from build123d import *

# Parameters (mm, degrees)
SKETCH1_W           = 47
SKETCH1_H           = 47
BOSS_EXTRUDE1_DEPTH = 30
SKETCH2_W           = 43.5
SKETCH2_H           = 43.5
CUT_EXTRUDE1_DEPTH  = 26.1
SKETCH5_W           = 47
SKETCH5_H           = 47
BOSS_EXTRUDE3_DEPTH = 3
CUT_EXTRUDE3_REACH  = 62.508
SKETCH4_W           = 2
SKETCH4_H           = 20
LPATTERN1_COUNT     = 7
LPATTERN1_PITCH     = 4
SKETCH8_W           = 26
SKETCH8_H           = 2
BOSS_EXTRUDE4_DEPTH = 2
LPATTERN2_COUNT     = 5
LPATTERN2_PITCH     = 4
SKETCH9_W           = 18
SKETCH9_H           = 9.389923451
CUT_EXTRUDE4_DEPTH  = 10
SKETCH10_W          = 15
SKETCH10_H          = 10
CUT_EXTRUDE5_DEPTH  = 61.508263898
SKETCH11_W          = 9.504801384
SKETCH11_H          = 14.465733587
SKETCH11_W_2        = 14.602344504
SKETCH11_H_2        = 6.519720082
CUT_EXTRUDE6_DEPTH  = 47.834816109


with BuildPart() as part:
    # Sketch1 → Boss-Extrude1 (new body)
    with BuildSketch(Plane(origin=(0, 0, 0), x_dir=(1, 0, 0), z_dir=(0, 1, 0))):
        Rectangle(SKETCH1_W, SKETCH1_H)
    extrude(amount=BOSS_EXTRUDE1_DEPTH)

    # Sketch2 → Cut-Extrude1 (cut)
    with BuildSketch(Plane.XZ):
        Rectangle(SKETCH2_W, SKETCH2_H)
    extrude(amount=-CUT_EXTRUDE1_DEPTH, mode=Mode.SUBTRACT)

    # Sketch5 → Boss-Extrude3 (add)
    with BuildSketch(Plane.XZ):
        Rectangle(SKETCH5_W, SKETCH5_H)
        Polygon((-16.6, 21.75), (-21.75, 21.75), (-21.75, 16.6), (-21.75, -16.6), (-21.75, -21.75), (-16.6, -21.75), (16.6, -21.75), (21.75, -21.75), (21.75, -16.6), (21.75, 16.6), (21.75, 21.75), (16.6, 21.75), align=None, mode=Mode.SUBTRACT)
    extrude(amount=BOSS_EXTRUDE3_DEPTH)

    # Sketch4 → Cut-Extrude3 (cut, up to next)
    with BuildSketch(Plane(origin=(0, 0, -23.5), x_dir=(-1, 0, 0), z_dir=(0, 0, -1)), mode=Mode.PRIVATE) as cut_extrude3_sk1:
        with Locations((-12, 13.157296847)):
            Rectangle(SKETCH4_W, SKETCH4_H)
    cut_extrude3_tool1 = extrude(cut_extrude3_sk1.sketch, amount=-CUT_EXTRUDE3_REACH, mode=Mode.PRIVATE) & part.part
    cut_extrude3 = cut_extrude3_tool1.solids().sort_by_distance((12, 13.157297, -23.5))[0]
    add(cut_extrude3, mode=Mode.SUBTRACT)

    # LPattern1: Cut-Extrude3 ×7
    with Locations(*[(-i * LPATTERN1_PITCH, 0, 0) for i in range(1, LPATTERN1_COUNT)]):
        add(cut_extrude3, mode=Mode.SUBTRACT)

    # Sketch8 → Boss-Extrude4 (add)
    with BuildSketch(Plane(origin=(0, 0, -23.5), x_dir=(-1, 0, 0), z_dir=(0, 0, -1))):
        with Locations((0, 20.157296847)):
            Rectangle(SKETCH8_W, SKETCH8_H)
    boss_extrude4 = extrude(amount=-BOSS_EXTRUDE4_DEPTH)

    # LPattern2: Boss-Extrude4 ×5
    with Locations(*[(0, -i * LPATTERN2_PITCH, 0) for i in range(1, LPATTERN2_COUNT)]):
        add(boss_extrude4)

    # Sketch9 → Cut-Extrude4 (cut)
    with BuildSketch(Plane.XY.offset(23.5)):
        with Locations((-9.5, 1.694961726)):
            Rectangle(SKETCH9_W, SKETCH9_H)
    extrude(amount=-CUT_EXTRUDE4_DEPTH, mode=Mode.SUBTRACT)

    # Sketch10 → Cut-Extrude5 (cut, through all)
    with BuildSketch(Plane.ZY.offset(23.5)):
        with Locations((6, 2)):
            Rectangle(SKETCH10_W, SKETCH10_H)
    extrude(amount=-CUT_EXTRUDE5_DEPTH, mode=Mode.SUBTRACT)

    # Sketch11 → Cut-Extrude6 (cut, through all)
    with BuildSketch(Plane(origin=(0, 30, 0), x_dir=(1, 0, 0), z_dir=(0, 1, 0))):
        with Locations((-15.948112, -5.914939324)):
            Rectangle(SKETCH11_W, SKETCH11_H)
        with Locations((-13.45587944, -18.519566616)):
            Rectangle(SKETCH11_W_2, SKETCH11_H_2)
        with Locations((15.948112, -5.914939324)):
            Rectangle(SKETCH11_W, SKETCH11_H)
        with Locations((13.45587944, -18.519566616)):
            Rectangle(SKETCH11_W_2, SKETCH11_H_2)
    extrude(amount=-CUT_EXTRUDE6_DEPTH, mode=Mode.SUBTRACT)


solid = part.part
Model file for the job. Use its own axes, mm. A direction names the side the tool comes from. Give positions to 0.01 mm unless a question says otherwise; leave off trailing zeros. Order: outer loops, then holes, each group sorted by start corner. A loop starts at its lowest first (then second) coordinate and runs counter-clockwise, first axis right, second up. Notation, with made-up numbers: M -9,67 L 37,67 A33 cw 37,96 Z; hole C 18.5,74.25 d7. An arc over 180 degrees is marked long. Put each result on its own line as item: value. Start each with the question number.
(1) Band-saw the part on A-A on x = 17.5. Give the cut face in (y, z), then the cut area to 3 significant figures.
(2) Band-saw the part on C-C on y = 2.5. Count the separate pieces of the cut face and the enclosed holes in it, then the cut area to 3 significant figures.
(3) Band-saw the part on B-B on z = 8.5. Give the cut face in (x, y).
(4) Pull direction Z, two halves, no side cores. Call faces 5 (the face through (9, 14, -23)), 6 (the face through (-20.757, 28, 19)): released by +Z, released by -Z, zero draft, split by the parting line, or undercut.
(5) Drill centre lines: L1, parallel to Z at x = 10.5, y = 18.5; L2, parallel to X at y = 13, z = -12; L3, parallel to X at y = 27, z = 17.5. Where is each one in solid material? Low to high. Write a range as [from, to].
(6) Pin check, flat tip, straight feed: pin 1 Ø12 at (x, z) = (-2.5, -7.5) entering from -Y. Stop position of the tip, or through.
(7) Tool access for faces 1 (the face through (-18.5, 2, 23)), 2 (the face through (6, 10, -21.75)), 3 (the face through (7, 18, -23)), 4 (the face through (14, -3, 22)): list every direction of +Z, -Z, +X, -X, +Y, -Y with a clear straight run to the whole face (end or side of a thin tool).
Results below:
1. outline: M -3,-23.5 L 30,-23.5 L 30,-1.32 L 26.1,-1.32 L 26.1,-21.75 L -3,-21.75 Z; M -3,21.78 L 30,21.78 L 30,23.5 L -3,23.5 Z; M 26.1,13.15 L 30,13.15 L 30,15.26 L 26.1,15.26 Z
1. area: 202 mm2
2. separate pieces: 3
2. enclosed holes: 0
2. area: 232 mm2
3. outline: M -23.5,7 L -21.75,7 L -21.75,26.1 L -20.7,26.1 L -20.7,30 L -23.5,30 Z; M -11.2,26.1 L 11.2,26.1 L 11.2,30 L -11.2,30 Z; M 20.7,26.1 L 21.75,26.1 L 21.75,7 L 23.5,7 L 23.5,30 L 20.7,30 Z
4. face 5: zero draft
4. face 6: undercut
5. L1: z = [-23.5, -21.75], [21.78, 23.5]
5. L2: x = [-23.5, -21.75], [21.75, 23.5]
5. L3: x = [-23.5, -20.76], [-6.15, 6.15], [20.76, 23.5]
6. pin 1: stops at y = 26.1
7. face 1: +Z, -Y
7. face 2: none
7. face 3: -Z
7. face 4: +Z, -Z, +X, -X, -Y
